Could you check a few things on this model? Use its own coordinates, in mm. A direction names the side the tool comes from. Round coordinates to 2 decimals unless told otherwise and drop trailing zeros. Loops run counter-clockwise (first coordinate to the right, second up) from the corner with the lowest first, then second, coordinate; pieces in that order, holes last. Notation, with made-up numbers: (-33, 52.5) -> (10, 52.5) arc R17 cw to (10, 84.5) -> close; hole circle Ø5 at (5, 82.25). An arc over 180 degrees is marked (long way). One line per item, written item: value.
```python
from build123d import *

# Parameters (mm, degrees)
SKETCH_1_W               = 42
SKETCH_1_H               = 42
EXTRUDE_1_DEPTH          = 10
SKETCH_2_R               = 21
EXTRUDE_2_DEPTH          = 45
SKETCH_3_R               = 4
EXTRUDE_3_DEPTH          = 18.5
CHAMFER_1_SIZE           = 4
SKETCH_4_R               = 11
CUT_EXTRUDE_1_DEPTH      = 25
SKETCH_5_R               = 12.5
EXTRUDE_4_DEPTH          = 2
CHAMFER_2_SIZE           = 1
SKETCH_6_R               = 2.1
CUT_EXTRUDE_2_DEPTH      = 2
PATTERN_CIRCULAR_1_COUNT = 4
SKETCH_7_R               = 2.1
CUT_EXTRUDE_3_DEPTH      = 8
PATTERN_CIRCULAR_2_COUNT = 4


with BuildPart() as part:
    # 草圖1 → 填料-伸長1 (new body)
    with BuildSketch(Plane(origin=(0, 0, 0), x_dir=(1, 0, 0), z_dir=(0, 1, 0))):
        Rectangle(SKETCH_1_W, SKETCH_1_H)
    extrude(amount=EXTRUDE_1_DEPTH)

    # 草圖2 → 填料-伸長2 (add)
    with BuildSketch(Plane(origin=(0, 10, 0), x_dir=(1, 0, 0), z_dir=(0, 1, 0))):
        Circle(SKETCH_2_R)
    extrude(amount=EXTRUDE_2_DEPTH)

    # 草圖3 → 填料-伸長3 (add)
    with BuildSketch(Plane(origin=(0, 55, 0), x_dir=(1, 0, 0), z_dir=(0, 1, 0))):
        Circle(SKETCH_3_R)
    extrude(amount=EXTRUDE_3_DEPTH)

    # 導角1
    chamfer_1_edges = [part.edges().sort_by_distance(p)[0] for p in [
        (21, 5, 21),
        (-21, 5, 21),
        (-21, 5, -21),
        (21, 5, -21),
    ]]
    chamfer(chamfer_1_edges, length=CHAMFER_1_SIZE)

    # 草圖4 → 除料-伸長1 (cut)
    with BuildSketch(Plane.XZ):
        Circle(SKETCH_4_R)
    extrude(amount=-CUT_EXTRUDE_1_DEPTH, mode=Mode.SUBTRACT)

    # 草圖5 → 填料-伸長4 (add)
    with BuildSketch(Plane(origin=(0, 55, 0), x_dir=(1, 0, 0), z_dir=(0, 1, 0))):
        Circle(SKETCH_5_R)
    extrude(amount=EXTRUDE_4_DEPTH)

    # 導角2
    chamfer_2_edges = [part.edges().sort_by_distance(p)[0] for p in [
        (-21, 55, 0),
    ]]
    chamfer(chamfer_2_edges, length=CHAMFER_2_SIZE)

    # 草圖6 → 除料-伸長2 (cut)
    with BuildSketch(Plane(origin=(0, 55, 0), x_dir=(1, 0, 0), z_dir=(0, 1, 0))):
        with Locations((-12.374368671, 12.374368671)):
            Circle(SKETCH_6_R)
    cut_extrude_2 = extrude(amount=-CUT_EXTRUDE_2_DEPTH, mode=Mode.SUBTRACT)

    # 環狀複製排列1: 除料-伸長2 ×4 about axis
    pattern_circular_1_axis = Axis((0, 0, 0), (0, 1, 0))
    for i in range(1, PATTERN_CIRCULAR_1_COUNT):
        add(cut_extrude_2.rotate(pattern_circular_1_axis, i * 360 / PATTERN_CIRCULAR_1_COUNT), mode=Mode.SUBTRACT)

    # 草圖7 → 除料-伸長3 (cut)
    with BuildSketch(Plane.XZ):
        with Locations((-15.5, 15.5)):
            Circle(SKETCH_7_R)
    cut_extrude_3 = extrude(amount=-CUT_EXTRUDE_3_DEPTH, mode=Mode.SUBTRACT)

    # 環狀複製排列2: 除料-伸長3 ×4 about axis
    pattern_circular_2_axis = Axis((0, 0, 0), (0, 1, 0))
    for i in range(1, PATTERN_CIRCULAR_2_COUNT):
        add(cut_extrude_3.rotate(pattern_circular_2_axis, i * 360 / PATTERN_CIRCULAR_2_COUNT), mode=Mode.SUBTRACT)


solid = part.part
```
Item 1: If we section it at B-B on y = 44.5: List the corners of the cut face in (x, z) for me.
Output:
outline: circle Ø42 at (0, 0)
Item 2: Will these pins go through, and if not, where does the flat tip stop? pin 1 Ø6.5 at (x, z) = (-5.5, 13.5) entering from +Y; pin 2 Ø1 at (x, y) = (-3.5, 24.5) entering from +Z; pin 3 Ø6.5 at (x, z) = (12.37, 12.37) entering from +Y.
Output:
pin 1: stops at y = 57
pin 2: stops at z = 20.78
pin 3: stops at y = 55
Item 3: I need wall thicknesses on line 1 (X direction, y = 4, z = -15); line 2 (X direction, y = 34.5, z = 0.5); line 3 (Y direction, x = -6, z = -16.5). Which ranges of each line are inside material? Lowest first, please. Write a range as from..to.
Output:
line 1: x = -21..-17.54, -13.46..13.46, 17.54..21
line 2: x = -20.99..20.99
line 3: y = 0..55
Item 4: For faces 4 (the face through (16, 10, 16)), 5 (the face through (16, 8, -16)), 6 (the face through (-21, 5, 0)), 7 (the face through (20.03, 31.69, -6.31)), 8 (the face through (16, 10, -16)), which set-ups out of +Z, -Z, +X, -X, +Y, -Y let a thin tool reach every point of the face, with its end or its side?
Output:
face 4: +Z, +X, +Y
face 5: -Y
face 6: +Z, -Z, -X, +Y, -Y
face 7: +Y
face 8: -Z, +X, +Y
Item 5: If we mould it in two halves opening along X, with no side actions, what happens to faces 1 (the face through (21, 5, 0)), 2 (the face through (10.371, 54.014, 13.005)), 3 (the face through (11.923, 55.986, -3.755))? For each: released by +X, released by -X, zero draft, split by the parting line, or undercut.
Output:
face 1: released by +X
face 2: undercut
face 3: split by the parting line
Item 6: If we section it at A-A on y = 11: List the corners of the cut face in (x, z) for me.
Output:
outline: circle Ø42 at (0, 0); hole circle Ø22 at (0, 0)
Item 7: If we section it at C-C on y = 69: List the corners of the cut face in (x, z) for me.
Output:
outline: circle Ø8 at (0, 0)
